The model under review builds one solid part; all positions refer to its coordinate system, in mm. Coordinates: 2 decimals unless noted, no trailing zeros. Order: outer loops, then holes, each group sorted by start corner. A loop starts at its lowest first (then second) coordinate and runs counter-clockwise, first axis right, second up. Notation, with made-up numbers: M 47.25,-4.5 L 89.25,-4.5 A27 ccw 89.25,30.5 Z; hole C 49,61.5 d8. An arc over 180 degrees is marked long. Answer as CSV lines item,"result". Start each with the question number.
Q1. For P1, Ø4, axis at x = 10, z = 7.5, coming from the -Y side, flat-tipped, find the tip position at first contact; note if it passes through.
Q2. Consider section C-C on y = -7. Write out the cut boundary in (x, z).
Q3. Consider section A-A on z = 7.5. Write out the cut boundary in (x, y), and give its area (3 significant figures).
Q4. Consider section B-B on x = 10. Write out the cut boundary in (y, z), and give its area (3 significant figures).
Q5. The part is to be moulded in two halves that separate along Z. For faces 1 (the face through (0, -5, 12.7)), 2 (the face through (-8.19, -5.07, 6.34)), 3 (the face through (-8.19, -5.07, -8.66)), 4 (the face through (-17, -5, 0)), say which applies: +Z half, -Z half, draft (parallel to the pull), parting line (faces both ways), or undercut.
Q6. Wall thickness on L1, parallel to X at y = -3.5, z = 7.5; L2, parallel to Z at x = 9, y = -4; L3, parallel to X at y = -8.5, z = 6.75: over which ranges is each line inside the solid? List them lowest first. Write a range as [from, to].
from build123d import *

# Parameters (mm, degrees)
SKETCH12_W           = 34
SKETCH12_H           = 25.4
BOSS_EXTRUDE2_DEPTH  = 10
M4_CLEARANCE_HOLE1_D = 4.3


with BuildPart() as part:
    # Sketch12 → Boss-Extrude2 (new body)
    with BuildSketch(Plane(origin=(0, 0, 0), x_dir=(1, 0, 0), z_dir=(0, 1, 0))):
        Rectangle(SKETCH12_W, SKETCH12_H)
    extrude(amount=-BOSS_EXTRUDE2_DEPTH)

    # M4 Clearance Hole1 (through all)
    with Locations(Plane(origin=(-10, 0, -7.5), x_dir=(0, 0, 1), z_dir=(0, 1, 0))):
        with Locations((0, 0), (15, 0), (15, 20), (0, 20)):
            Hole(M4_CLEARANCE_HOLE1_D / 2)


solid = part.part
Evaluation:
1,P1,"passes through"
2,outline,"M -17,-12.7 L 17,-12.7 L 17,12.7 L -17,12.7 Z; hole C -10,-7.5 d4.3; hole C -10,7.5 d4.3; hole C 10,-7.5 d4.3; hole C 10,7.5 d4.3"
3,outline,"M -17,-10 L -12.15,-10 L -12.15,0 L -17,0 Z; M -7.85,-10 L 7.85,-10 L 7.85,0 L -7.85,0 Z; M 12.15,-10 L 17,-10 L 17,0 L 12.15,0 Z"
3,area,"254 mm²"
4,outline,"M -10,-12.7 L 0,-12.7 L 0,-9.65 L -10,-9.65 Z; M -10,-5.35 L 0,-5.35 L 0,5.35 L -10,5.35 Z; M -10,9.65 L 0,9.65 L 0,12.7 L -10,12.7 Z"
4,area,"168 mm²"
5,face 1,"+Z half"
5,face 2,"undercut"
5,face 3,"undercut"
5,face 4,"draft"
6,L1,"x = [-17, -12.15], [-7.85, 7.85], [12.15, 17]"
6,L2,"z = [-12.7, -9.4], [-5.6, 5.6], [9.4, 12.7]"
6,L3,"x = [-17, -12.01], [-7.99, 7.99], [12.01, 17]"
